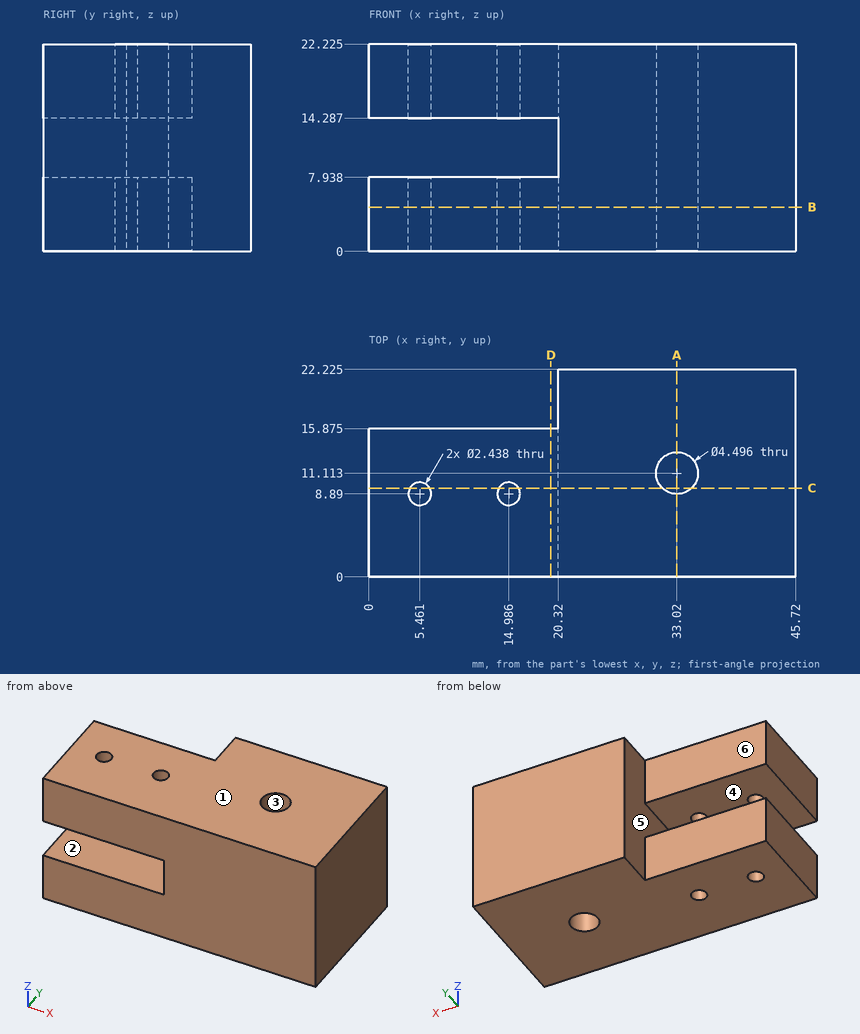
Drawing for the job (mm, zero at the part's lowest x, y, z). A direction names the side the tool comes from. Give positions to 0.01 mm unless a question says otherwise; leave off trailing zeros. Order: outer loops, then holes, each group sorted by start corner. A loop starts at its lowest first (then second) coordinate and runs counter-clockwise, first axis right, second up. Notation, with made-up numbers: M 43,65.25 L 89,65.25 A15 ccw 89,77.25 Z; hole C -8,-24.5 d4. An arc over 180 degrees is marked long. Use a Markdown table: item, result. Add a question column.
(1) Drop flat-ended pins along their axis: P1, Ø4, axis at x = 31, z = 7, coming from the -Y side; P2, Ø2, axis at x = 5.461, y = 8.89, coming from the -Z side; P3, Ø6.5, axis at x = 15, z = 16.5, coming from the +Y side (1 decimal). Give the stop position or say it passes through.
(2) Mould opens along Z. For the marked faces 1, 2 and 3 say: +Z half, -Z half, draft (parallel to the pull), parting line (faces both ways), or undercut.
(3) Saw through at D-D, the plane x = 19.5. Give the cut face in (y, z) (1 decimal).
(4) Saw through at B-B, the plane z = 4.75. Give the cut face in (x, y) (1 decimal).
(5) 3-axis set-ups, long thin cutter, end or side, ignore diameter. For the marked faces 4, 5 and 6: which of +Z, -Z, +X, -X, +Y, -Y reach the whole face in a straight line?
(6) Saw through at A-A, the plane x = 33.02. Give the cut face in (y, z) (1 decimal).
(7) Saw through at C-C, the plane y = 9.5. Give the cut face in (x, z) (1 decimal).
(8) Probe line 1 along Y through (x, z) = (33.02, 7.75) (1 decimal); line 2 along Z through (x, y) = (16.5, 11.5) (1 decimal); line 3 along X through (y, z) = (20, 9.5). List the from-to ranges inside material, lowest first. Write a range as [from, to].
Answer key:
| question | item | result |
|---|---|---|
| 1 | P1 | y = 0 |
| 1 | P2 | through |
| 1 | P3 | y = 15.9 |
| 2 | face 1 | +Z half |
| 2 | face 2 | undercut |
| 2 | face 3 | draft |
| 3 | outline | M 0,0 L 15.9,0 L 15.9,7.9 L 0,7.9 Z; M 0,14.3 L 15.9,14.3 L 15.9,22.2 L 0,22.2 Z |
| 4 | outline | M 0,0 L 45.7,0 L 45.7,22.2 L 20.3,22.2 L 20.3,15.9 L 0,15.9 Z; hole C 5.5,8.9 d2.4; hole C 15,8.9 d2.4; hole C 33,11.1 d4.5 |
| 5 | face 4 | -X, +Y, -Y |
| 5 | face 5 | -X, +Y |
| 5 | face 6 | +Z, -Z, -X, +Y |
| 6 | outline | M 0,0 L 8.9,0 L 8.9,22.2 L 0,22.2 Z; M 13.4,0 L 22.2,0 L 22.2,22.2 L 13.4,22.2 Z |
| 7 | outline | M 0,0 L 4.4,0 L 4.4,7.9 L 0,7.9 Z; M 0,14.3 L 4.4,14.3 L 4.4,22.2 L 0,22.2 Z; M 6.5,0 L 13.9,0 L 13.9,7.9 L 6.5,7.9 Z; M 6.5,14.3 L 13.9,14.3 L 13.9,22.2 L 6.5,22.2 Z; M 16,0 L 31.5,0 L 31.5,22.2 L 16,22.2 L 16,14.3 L 20.3,14.3 L 20.3,7.9 L 16,7.9 Z; M 34.6,0 L 45.7,0 L 45.7,22.2 L 34.6,22.2 Z |
| 8 | line 1 | [0, 8.9], [13.4, 22.2] |
| 8 | line 2 | [0, 7.9], [14.3, 22.2] |
| 8 | line 3 | [20.32, 45.72] |
